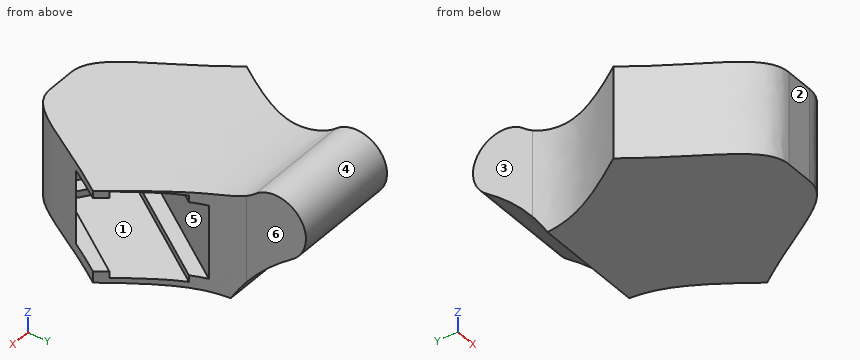
```python
from build123d import *

# Parameters (mm, degrees)
BOSS_EXTRUDE1_DEPTH      = 70
BOSS_EXTRUDE1_DEPTH_BACK = 90
CUT_EXTRUDE1_DEPTH       = 125.755860093
CUT_EXTRUDE1_DEPTH_BACK  = 125.755860093
SKETCH10_OUTSIDE_W       = 205.76
SKETCH10_OUTSIDE_H       = 165.428
CUT_EXTRUDE4_DEPTH       = 6.4
CUT_EXTRUDE4_DEPTH_BACK  = 105.067072527
SKETCH15_W               = 36.6
SKETCH15_H               = 30.6
CUT_EXTRUDE5_DEPTH       = 12.5


with BuildPart() as part:
    # Sketch8 → Boss-Extrude1 (new, two sides: drawn at the far end of the back side and taken through both)
    with BuildSketch(Plane.XY.offset(-BOSS_EXTRUDE1_DEPTH_BACK)):
        with BuildLine():
            Line((-6, -45.667592609), (6, -45.667592609))
            add(Edge.make_bspline(
                [(44.587269323, 0), (24.684424598, -27.160649005), (19.273508518, -45.667592609), (6, -45.667592609)],
                knots=[0, 0, 0, 0, 1, 1, 1, 1], degree=3))
            add(Edge.make_bspline(
                [(23.5, 49), (23.5, 34.38564976), (25.853420885, 25.6357926), (44.587269323, 0)],
                knots=[0, 0, 0, 0, 1, 1, 1, 1], degree=3))
            Line((23.5, 49), (23.5, 74))
            Line((23.5, 74), (-23.5, 74))
            Line((-23.5, 74), (-23.5, 49))
            add(Edge.make_bspline(
                [(-23.5, 49), (-23.5, 34.38564976), (-25.853420885, 25.6357926), (-44.587269323, 0)],
                knots=[0, 0, 0, 0, 1, 1, 1, 1], degree=3))
            add(Edge.make_bspline(
                [(-44.587269323, 0), (-24.684424598, -27.160649005), (-19.273508518, -45.667592609), (-6, -45.667592609)],
                knots=[0, 0, 0, 0, 1, 1, 1, 1], degree=3))
        make_face()
    extrude(amount=BOSS_EXTRUDE1_DEPTH + BOSS_EXTRUDE1_DEPTH_BACK)

    # Sketch10 outside → Cut-Extrude1 (cut, two sides: drawn at the far end of the back side and taken through both)
    with BuildSketch(Plane(origin=(0, 0, 0), x_dir=(0, 0, -1), z_dir=(1, 0, 0)).offset(-CUT_EXTRUDE1_DEPTH_BACK)):
        with Locations((10, 14.166)):
            Rectangle(SKETCH10_OUTSIDE_W, SKETCH10_OUTSIDE_H)
        with BuildLine():
            Line((19.25, -45.667592609), (20.75, 42.667592609))
            add(Edge.make_bspline(
                [(-6.284762028, 68.360956134), (4.979548326, 51.963661564), (20.75, 42.667592609)],
                knots=[0, 0, 0, 1, 1, 1], degree=2))
            ThreePointArc((-6.284762028, 68.360956134), (-24.867699079, 71.348879707), (-26.958577761, 52.643761074))
            add(Edge.make_bspline(
                [(-26.958577761, 52.643761074), (-14.483902489, 37.777022003), (-19.25, -11.054872301), (-19.25, -45.667592609)],
                knots=[0, 0, 0, 0, 1, 1, 1, 1], degree=3))
            Line((-19.25, -45.667592609), (19.25, -45.667592609))
        make_face(mode=Mode.SUBTRACT)
    extrude(amount=CUT_EXTRUDE1_DEPTH + CUT_EXTRUDE1_DEPTH_BACK, mode=Mode.SUBTRACT)

    # l_hip_x_top_room → Cut-Extrude4 (cut, two sides: drawn at the far end of the back side and taken through both)
    with BuildSketch(Plane(origin=(-7.847220638, -10.738301926, 0), x_dir=(-0.807391122257892, 0.5900165893423182, 0), z_dir=(-0.5900165893423182, -0.807391122257892, 0)).offset(-CUT_EXTRUDE4_DEPTH_BACK)):
        Polygon((-5.7, 15.3), (0.1, 15.3), (0.1, -15.3), (-5.7, -15.3), (-5.7, -18.05), (-30.7, -18.05), (-30.7, -15.3), (-36.5, -15.3), (-36.5, 15.3), (-30.7, 15.3), (-30.7, 18.05), (-5.7, 18.05), align=None)
    extrude(amount=CUT_EXTRUDE4_DEPTH + CUT_EXTRUDE4_DEPTH_BACK, mode=Mode.SUBTRACT)

    # Sketch15 → Cut-Extrude5 (cut)
    with BuildSketch(Plane(origin=(-7.847220638, -10.738301926, 0), x_dir=(0.807391122257892, -0.5900165893423182, 0), z_dir=(0.5900165893423182, 0.807391122257892, 0))):
        with Locations((18.2, 0)):
            Rectangle(SKETCH15_W, SKETCH15_H)
    extrude(amount=-CUT_EXTRUDE5_DEPTH, mode=Mode.SUBTRACT)


solid = part.part
```
The listing builds one solid part. Answer for the finished solid, in the listing's coordinates (mm). Face numbers are marked on the shaded views. A direction names the side the tool comes from. Give positions to 0.01 mm unless a question says otherwise; leave off trailing zeros. Use one line per item in the form item = value. Start each with the question number.
1) The mould has two halves that part along Y. Classify the marked faces 4, 5 and 6: pulls with the +Y half, pulls with the -Y half, needs draft (parallel to the pull), parting line crosses it, or undercut.
2) A tool of negligible diameter and unlimited length cuts with its end or side. For the marked faces 1, 2 and 3, from which of +Z, -Z, +X, -X, +Y, -Y can it reach the whole face along a straight path? Write none if from no direction.
3) Consider line 1 along Y through (x, z) = (-13, -14); line 2 along Z through (x, y) = (14, -29); line 3 along Y through (x, z) = (-15, -4). Determine where each line is inside the solid, lowest interval first. Write a range as from..to.
4) Flat-ended cylindrical pins translate along their axes: pin 1 Ø6 at (x, y) = (-26, 55.5) entering from +Z; pin 2 Ø1 at (x, y) = (3, -1) entering from +Z; pin 3 Ø3 at (y, z) = (-20, -10) entering from +X; pin 4 Ø6 at (x, z) = (18.5, 17.5) entering from +Y. Find the tip coordinate at first contact, or state that the pin passes through.
Geometry results:
q1.face_4 = parting line crosses it
q1.face_5 = undercut
q1.face_6 = needs draft
q2.face_1 = none
q2.face_2 = +Z, -Z, +X, -X, -Y
q2.face_3 = +Z, -Z, -X, +Y
q3.line_1 = -43.65..-22.45, -17.62..47.12
q3.line_2 = -19.53..-18.05, 18.05..19
q3.line_3 = -42.21..-20.99, -20.36..55.81
q4.pin_1 = 29.42
q4.pin_2 = 18.38
q4.pin_3 = 32.09
q4.pin_4 = 74
